from build123d import *

# Parameters (mm, degrees)
BOSS_EXTRUDE1_DEPTH = 3.175


with BuildPart() as part:
    # Sketch1 → Boss-Extrude1 (new body)
    with BuildSketch(Plane(origin=(0, 0, 0), x_dir=(1, 0, 0), z_dir=(0, 1, 0))):
        with BuildLine():
            Line((-10.25, 11.6), (-10.25, 31.683236893))
            ThreePointArc((-10.25, 31.683236893), (-19.590367531, -26.927820187), (33.3, 0))
            ThreePointArc((33.3, 0), (26.927820187, 19.590367531), (10.25, 31.683236893))
            Line((10.25, 31.683236893), (10.25, 11.6))
            Line((10.25, 11.6), (10.490250515, 0.452376089))
            ThreePointArc((10.490250515, 0.452376089), (10.497562346, 0.226240568), (10.5, 0))
            ThreePointArc((10.5, 0), (0, -10.5), (-10.5, 0))
            ThreePointArc((-10.5, 0), (-10.497562346, 0.226240568), (-10.490250515, 0.452376089))
            Line((-10.490250515, 0.452376089), (-10.25, 11.6))
        make_face()
    extrude(amount=BOSS_EXTRUDE1_DEPTH)


solid = part.part
Source: CAD feature listing. Evaluate the final solid. Frame: model axes, mm. A direction names the side the tool comes from. Give positions to 0.01 mm unless a question says otherwise; leave off trailing zeros. Loops run counter-clockwise (first coordinate to the right, second up) from the corner with the lowest first, then second, coordinate; pieces in that order, holes last. Notation, with made-up numbers: (68, 72) -> (90, 72) arc R34 cw to (90, 110) -> close; hole circle Ø7 at (19, 26.5). An arc over 180 degrees is marked (long way). Use a Markdown table: item, result. Add a question column.
1) Section query B-B, the plane y = 1.1. Return the cut outline in (x, z), then the cut area to 3 significant figures.
2) Reachability of faces 1 (the face through (-8, 0, 8)), 2 (the face through (10.25, 2, -22)) from +Z, -Z, +X, -X, +Y, -Y: full face, straight path, thin tool, end or side. Return the list, or none.
3) Section query D-D, the plane x = 0. Return the cut outline in (y, z) (3 decimals).
4) Line query: line 1 along X through (y, z) = (0.75, -1); line 2 along X through (y, z) = (0.75, 2); line 3 along X through (y, z) = (1.7, 13). Output: solid intervals per line, ascending. Write a range as [from, to].
5) Section query A-A, the plane z = -25.5. Return the cut outline in (x, y) (3 decimals), then the cut area to 3 significant figures.
6) Section query C-C, the plane z = -7. Return the cut outline in (x, y) (3 decimals), then the cut area to 3 significant figures.
7) First-contact query: pin 1 (1.6 mm diameter, centred on y = 1, z = -21, fed in from +X); pin 2 (1.5 mm diameter, centred on y = 1, z = 2.5, fed in from -X). Flat tips, straight axial feed; report the tip coordinate or a pass-through.
Numbers:
| question | item | result |
|---|---|---|
| 1 | outline | (-10.5, 0) arc R10.5 cw to (10.5, 0) arc R10.5 cw to (10.49, -0.45) -> (10.25, -11.6) -> (10.25, -31.68) arc R33.3 ccw (long way) to (-10.25, -31.68) -> (-10.25, -11.6) -> (-10.49, -0.45) arc R10.5 cw to start |
| 1 | area | 2,640 mm2 |
| 2 | face 1 | +Z, -Z, +X, -X, -Y |
| 2 | face 2 | -Z, +Y, -Y |
| 3 | outline | (0, 10.5) -> (3.175, 10.5) -> (3.175, 33.3) -> (0, 33.3) -> close |
| 4 | line 1 | x = [-33.28, -10.48], [10.48, 33.28] |
| 4 | line 2 | x = [-33.24, -10.31], [10.31, 33.24] |
| 4 | line 3 | x = [-30.66, 30.66] |
| 5 | outline | (-21.416, 0) -> (-10.25, 0) -> (-10.25, 3.175) -> (-21.416, 3.175) -> close; (10.25, 0) -> (21.416, 0) -> (21.416, 3.175) -> (10.25, 3.175) -> close |
| 5 | area | 70.9 mm2 |
| 6 | outline | (-32.556, 0) -> (-10.349, 0) -> (-10.349, 3.175) -> (-32.556, 3.175) -> close; (10.349, 0) -> (32.556, 0) -> (32.556, 3.175) -> (10.349, 3.175) -> close |
| 6 | area | 141 mm2 |
| 7 | pin 1 | stops at x = 26.47 |
| 7 | pin 2 | stops at x = -33.25 |
